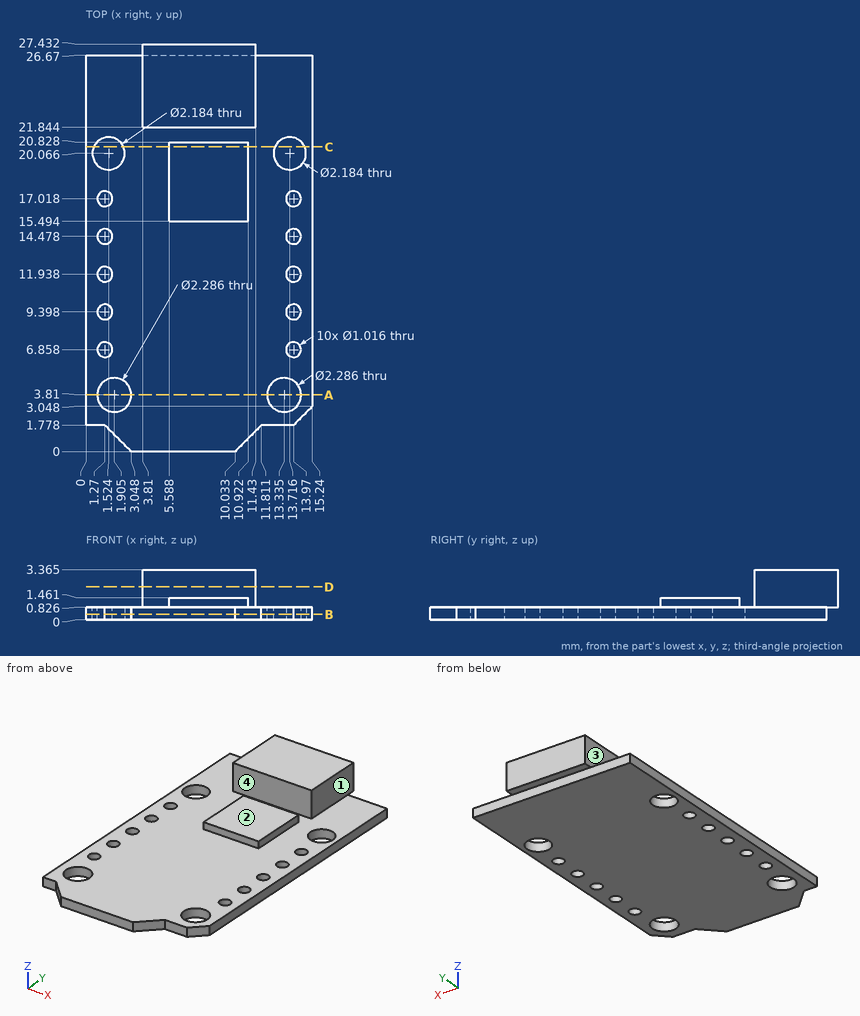
Geometry check sheet. Reference: drawing and pictorial views, mm from the part's lowest x, y, z. A direction names the side the tool comes from. Coordinates: 2 decimals unless noted, no trailing zeros. Loops run counter-clockwise (first coordinate to the right, second up) from the corner with the lowest first, then second, coordinate; pieces in that order, holes last. Notation, with made-up numbers: M 23,22.5 L 45,22.5 A20 ccw 45,39.5 Z; hole C -2.75,5.25 d9. An arc over 180 degrees is marked long. One line per item, written item: value.
1. Section check B-B on z = 0.35. Give the number of separate pieces and of enclosed holes in the cut face, plus the area to 3 significant figures.
Answers follow:
separate pieces: 1
enclosed holes: 14
area: 370 mm^2
2. Section check D-D on z = 2.2. Record the cut outline in (x, y) (1 decimal).
Answers follow:
outline: M 3.8,21.8 L 11.4,21.8 L 11.4,27.4 L 3.8,27.4 Z
3. Material ranges on line 1 along Y through (x, z) = (6.5, 1) (1 decimal); line 2 along X through (y, z) = (4, 0.7); line 3 along Z through (x, y) = (4.5, 6.25) (1 decimal), recorded low to high. Write a range as from..to.
Answers follow:
line 1: 15.5..20.8, 21.8..27.4
line 2: 0..0.78, 3.03..12.21, 14.46..15.24
line 3: 0..0.8
4. Section check A-A on y = 3.81. Record the cut outline in (x, z) (1 decimal).
Answers follow:
outline: M 0,0 L 0.8,0 L 0.8,0.8 L 0,0.8 Z; M 3,0 L 12.2,0 L 12.2,0.8 L 3,0.8 Z; M 14.5,0 L 15.2,0 L 15.2,0.8 L 14.5,0.8 Z
5. Section check C-C on y = 20.5. Record the cut outline in (x, z) (1 decimal).
Answers follow:
outline: M 0,0 L 0.5,0 L 0.5,0.8 L 0,0.8 Z; M 2.5,0 L 12.7,0 L 12.7,0.8 L 10.9,0.8 L 10.9,1.5 L 5.6,1.5 L 5.6,0.8 L 2.5,0.8 Z; M 14.7,0 L 15.2,0 L 15.2,0.8 L 14.7,0.8 Z
6. Gauge pin test, flat ends, axial feed: P1, Ø5, axis at x = 11.5, y = 13, coming from the +Z side (1 decimal); P2, Ø1.3, axis at y = 25.5, z = 2, coming from the -X side; P3, Ø0.6, axis at x = 13.97, y = 11.938, coming from the -Z side. Record the tip position at first contact, or that the pin passes through.
Answers follow:
P1: z = 0.8
P2: x = 3.81
P3: through
7. Set-up check for the marked faces 1, 2, 3 and 4: record each of +Z, -Z, +X, -X, +Y, -Y from which the full face is reachable in a straight line by a thin tool's end or side.
Answers follow:
face 1: +Z, +X, +Y, -Y
face 2: +Z, +X, -X, -Y
face 3: +Z, -X, +Y, -Y
face 4: +Z, +X, -X
